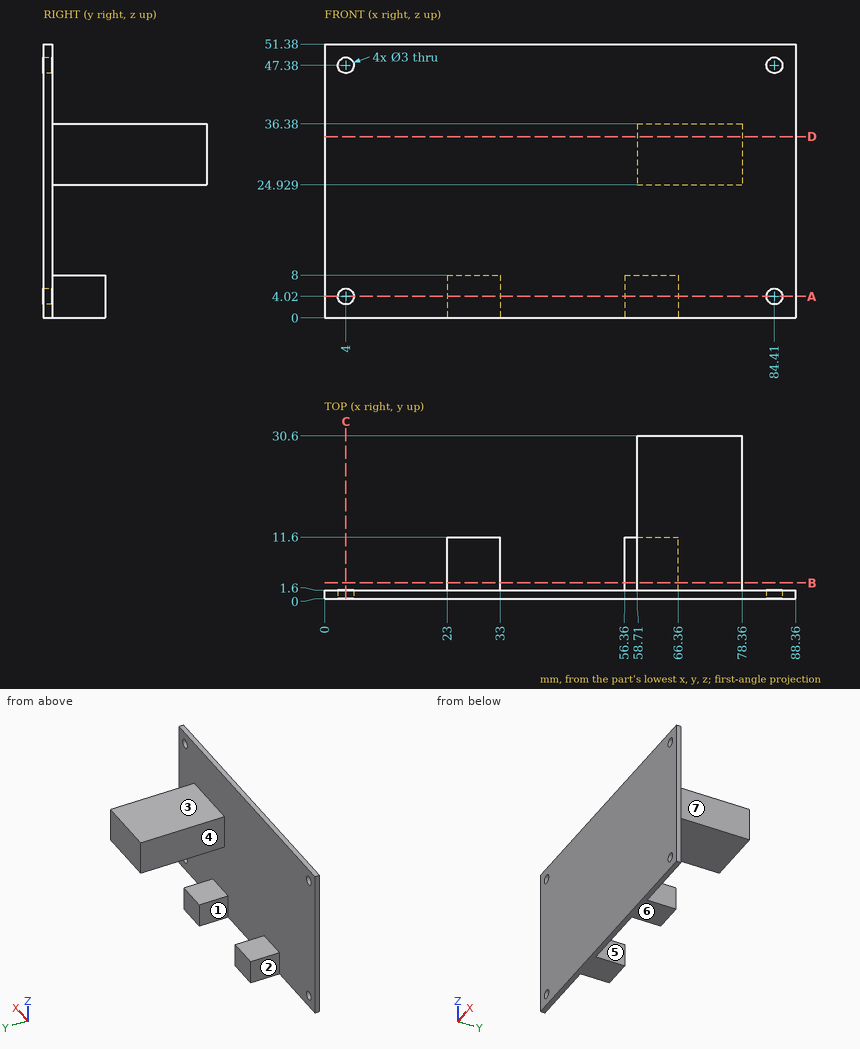
Can you work these out from the drawing? Everything is in mm from the part's minimum corner. A direction names the side the tool comes from. Round coordinates to 2 decimals unless told otherwise and drop trailing zeros. Write each loop counter-clockwise with the first axis right and the second up, starting at its lowest first coordinate (ties: lowest second). Pieces come first, ordered by that corner, then holes. Notation, with made-up numbers: M 85.25,89.25 L 93.25,89.25 A34 ccw 93.25,123.25 Z; hole C 14.25,-1.75 d1. An arc over 180 degrees is marked long. Use a Markdown table: item, result.
Item 1: I want a section at B-B (y = 3). List the corners of the cut face in (x, z) for me.
Found:
| item | result |
|---|---|
| outline | M 23,0 L 33,0 L 33,8 L 23,8 Z; M 56.36,0 L 66.36,0 L 66.36,8 L 56.36,8 Z; M 58.71,24.93 L 78.36,24.93 L 78.36,36.38 L 58.71,36.38 Z |
Item 2: I want a section at C-C (x = 4). List the corners of the cut face in (y, z) for me.
Found:
| item | result |
|---|---|
| outline | M 0,0 L 1.6,0 L 1.6,2.52 L 0,2.52 Z; M 0,5.52 L 1.6,5.52 L 1.6,45.88 L 0,45.88 Z; M 0,48.88 L 1.6,48.88 L 1.6,51.38 L 0,51.38 Z |
Item 3: We'd pull the mould along X, two halves only. Please class the marked faces 4, 5, 6 and 7: released by +X, released by -X, zero draft, split by the parting line, or undercut.
Found:
| item | result |
|---|---|
| face 4 | released by -X |
| face 5 | undercut |
| face 6 | zero draft |
| face 7 | released by +X |
Item 4: I want a section at A-A (z = 4.02). List the corners of the cut face in (x, y) for me.
Found:
| item | result |
|---|---|
| outline | M 0,0 L 2.5,0 L 2.5,1.6 L 0,1.6 Z; M 5.5,0 L 82.91,0 L 82.91,1.6 L 66.36,1.6 L 66.36,11.6 L 56.36,11.6 L 56.36,1.6 L 33,1.6 L 33,11.6 L 23,11.6 L 23,1.6 L 5.5,1.6 Z; M 85.91,0 L 88.36,0 L 88.36,1.6 L 85.91,1.6 Z |
Item 5: I want a section at D-D (z = 34). List the corners of the cut face in (x, y) for me, and give its area (3 significant figures).
Found:
| item | result |
|---|---|
| outline | M 0,0 L 88.36,0 L 88.36,1.6 L 78.36,1.6 L 78.36,30.6 L 58.71,30.6 L 58.71,1.6 L 0,1.6 Z |
| area | 711 mm2 |
Item 6: Which directions (+Z, -Z, +X, -X, +Y, -Y) give clear straight access to the entire face, cutting with the end or side of a thin tool? Please do the marked faces 1, 2 and 3.
Found:
| item | result |
|---|---|
| face 1 | +Z, -Z, +Y |
| face 2 | +Z, -Z, -X, +Y |
| face 3 | +Z, +X, -X, +Y |
Item 7: If I drill on line 1 along X through (y, z) = (0.45, 4.02); line 2 along Z through (x, y) = (84, 1); line 3 along Y through (x, z) = (12, 11), over which ranges is the centre line in solid material (lowest first)? Write a range as [from, to].
Found:
| item | result |
|---|---|
| line 1 | x = [0, 2.5], [5.5, 82.91], [85.91, 88.36] |
| line 2 | z = [0, 2.58], [5.46, 45.94], [48.82, 51.38] |
| line 3 | y = [0, 1.6] |
Item 8: For pin 1 Ø9 at (x, z) = (28.5, 3.5) entering from +Y; pin 2 Ø4 at (x, z) = (4, 47.38) entering from +Y; pin 3 Ø6 at (x, y) = (67.5, 10.5) entering from +Z; pin 4 Ø2.5 at (x, z) = (84.41, 4.02) entering from -Y, each with a flat end and sliding along its axis, tell me the tip position at first contact or that it passes through.
Found:
| item | result |
|---|---|
| pin 1 | stops at y = 11.6 |
| pin 2 | stops at y = 1.6 |
| pin 3 | stops at z = 36.38 |
| pin 4 | passes through |
